from build123d import *

# Parameters (mm, degrees)
BOSS_EXTRUDE1_DEPTH = 654.07286
CUT_EXTRUDE1_REACH  = 5.175
SKETCH2_R           = 2.54


with BuildPart() as part:
    # Sketch1 → Boss-Extrude1 (new body)
    with BuildSketch(Plane(origin=(0, 0, 0), x_dir=(0, 0, -1), z_dir=(1, 0, 0))):
        with BuildLine():
            Line((3.175, 3.175), (16.51, 3.175))
            ThreePointArc((16.51, 3.175), (18.306051224, 2.431051224), (19.05, 0.635))
            Line((19.05, 0.635), (19.05, 0))
            Line((19.05, 0), (0, 0))
            Line((0, 0), (0, 19.05))
            Line((0, 19.05), (0.635, 19.05))
            ThreePointArc((0.635, 19.05), (2.431051224, 18.306051224), (3.175, 16.51))
            Line((3.175, 16.51), (3.175, 3.175))
        make_face()
    extrude(amount=BOSS_EXTRUDE1_DEPTH)

    # Sketch2 → Cut-Extrude1 (cut, up to next)
    with BuildSketch(Plane(origin=(0, 3.175, 0), x_dir=(1, 0, 0), z_dir=(0, 1, 0)), mode=Mode.PRIVATE) as cut_extrude1_sk1:
        with Locations((641.37286, 9.8425)):
            Circle(SKETCH2_R)
    cut_extrude1_tool1 = extrude(cut_extrude1_sk1.sketch, amount=-CUT_EXTRUDE1_REACH, mode=Mode.PRIVATE) & part.part
    add(cut_extrude1_tool1.solids().sort_by_distance((641.37286, 3.175, -9.8425))[0], mode=Mode.SUBTRACT)
    # Sketch2 → Cut-Extrude1 (cut, up to next)
    with BuildSketch(Plane(origin=(0, 3.175, 0), x_dir=(1, 0, 0), z_dir=(0, 1, 0)), mode=Mode.PRIVATE) as cut_extrude1_sk2:
        with Locations((12.7, 9.8425)):
            Circle(SKETCH2_R)
    cut_extrude1_tool2 = extrude(cut_extrude1_sk2.sketch, amount=-CUT_EXTRUDE1_REACH, mode=Mode.PRIVATE) & part.part
    add(cut_extrude1_tool2.solids().sort_by_distance((12.7, 3.175, -9.8425))[0], mode=Mode.SUBTRACT)


solid = part.part
For this review, take the finished solid that the model builds, in its own axes (mm). A direction names the side the tool comes from. Round coordinates to 2 decimals unless told otherwise and drop trailing zeros. Write each loop counter-clockwise with the first axis right and the second up, starting at its lowest first coordinate (ties: lowest second). Pieces come first, ordered by that corner, then holes. Notation, with made-up numbers: (88.5, 8) -> (108.5, 8) arc R26 cw to (108.5, 23) -> close; hole circle Ø1 at (46.25, 0.5). An arc over 180 degrees is marked (long way). Use CSV: the item, a comma, the result in double quotes.
(1) Consider section B-B, the plane y = 9. Give the boundary of the cut face in (x, z) (3 decimals).
Computed values:
outline,"(0, -3.175) -> (654.073, -3.175) -> (654.073, 0) -> (0, 0) -> close"
(2) Clearance check with flat-ended pins moving along their axes: P1, Ø4, axis at x = 280.5, z = -10.5, coming from the +Y side (3 decimals); P2, Ø3, axis at x = 641.37, z = -9.84, coming from the +Y side; P3, Ø2, axis at x = 173, y = 9.5, coming from the -Z side (3 decimals). State where each tip first meets the part, or that it passes through.
Computed values:
P1,"y = 3.175"
P2,"through"
P3,"z = -3.175"
(3) Consider section A-A, the plane x = 346. Give the boundary of the cut face in (y, z) (3 decimals), plus the area to 3 significant figures.
Computed values:
outline,"(0, -19.05) -> (0.635, -19.05) arc R2.54 ccw to (3.175, -16.51) -> (3.175, -3.175) -> (16.51, -3.175) arc R2.54 ccw to (19.05, -0.635) -> (19.05, 0) -> (0, 0) -> close"
area,"108 mm²"
(4) For faces 1 (the face through (322, 0, -10)), 2 (the face through (322, 3.175, -10)), list the 3-axis set-ups (+Z, -Z, +X, -X, +Y, -Y) from which the entire face can be reached by the end or side of a thin tool; tool diameter is ignored.
Computed values:
face 1,"+Z, -Z, +X, -X, -Y"
face 2,"-Z, +X, -X, +Y"
(5) To check wall thickness, follow L1, parallel to Z at x = 12.7, y = 1.35; L2, parallel to Y at x = 350, z = -12 (3 decimals); L3, parallel to Z at x = 56.5, y = 6 (3 decimals). State the ranges of each line that lie inside material, in increasing order. Write a range as [from, to].
Computed values:
L1,"[-18.95, -12.38], [-7.3, 0]"
L2,"[0, 3.175]"
L3,"[-3.175, 0]"
